from build123d import *

# Parameters (mm, degrees)
SKETCH1_W                    = 12
SKETCH1_H                    = 40
BOSS_EXTRUDE1_DEPTH          = 600
FILLET1_R                    = 12
SKETCH2_W                    = 1150
SKETCH2_H                    = 12
CUT_EXTRUDE1_DEPTH           = 2
FILLET2_R                    = 5
CUT_EXTRUDE2_REACH           = 14
SKETCH3_R                    = 4
F_4_0_4_DIAMETER_HOLE1_D     = 4
F_4_0_4_DIAMETER_HOLE1_DEPTH = 10
LPATTERN1_COUNT              = 4
LPATTERN1_PITCH              = 350
SKETCH6_W                    = 15
SKETCH6_H                    = 16
BOSS_EXTRUDE2_DEPTH          = 12
CUT_EXTRUDE6_REACH           = 17
SKETCH7_W                    = 2
SKETCH7_H                    = 12
FILLET3_R                    = 3


with BuildPart() as part:
    # Sketch1 → Boss-Extrude1 (new body, symmetric)
    with BuildSketch(Plane.XY):
        Rectangle(SKETCH1_W, SKETCH1_H)
    extrude(amount=BOSS_EXTRUDE1_DEPTH, both=True)

    # Fillet1
    fillet1_edges = [part.edges().sort_by_distance(p)[0] for p in [
        (0, -20, 600),
        (0, -20, -600),
        (0, 20, -600),
        (0, 20, 600),
    ]]
    fillet(fillet1_edges, radius=FILLET1_R)

    # Sketch2 → Cut-Extrude1 (cut)
    with BuildSketch(Plane(origin=(6, 0, 0), x_dir=(0, 0, -1), z_dir=(1, 0, 0))):
        with Locations((-25, 0)):
            Rectangle(SKETCH2_W, SKETCH2_H)
    extrude(amount=-CUT_EXTRUDE1_DEPTH, mode=Mode.SUBTRACT)

    # Fillet2
    fillet2_edges = [part.edges().sort_by_distance(p)[0] for p in [
        (5, 6, -550),
        (5, -6, -550),
    ]]
    fillet(fillet2_edges, radius=FILLET2_R)

    # Sketch3 → Cut-Extrude2 (cut, up to next)
    with BuildSketch(Plane(origin=(6, 0, 0), x_dir=(0, 0, -1), z_dir=(1, 0, 0)), mode=Mode.PRIVATE) as cut_extrude2_sk1:
        with Locations(Location((590, 0, 0), (0, 0, 90))):  # turned: the seam where the file's is
            Circle(SKETCH3_R)
    cut_extrude2_tool1 = extrude(cut_extrude2_sk1.sketch, amount=-CUT_EXTRUDE2_REACH, mode=Mode.PRIVATE) & part.part
    add(cut_extrude2_tool1.solids().sort_by_distance((6, 0, -590))[0], mode=Mode.SUBTRACT)

    # Ø4.0 (4) Diameter Hole1
    with Locations(Plane.ZY.offset(6)):
        with Locations((570, 0)):
            f_4_0_4_diameter_hole1 = Hole(F_4_0_4_DIAMETER_HOLE1_D / 2, depth=F_4_0_4_DIAMETER_HOLE1_DEPTH)

    # LPattern1: Ø4.0 (4) Diameter Hole1 ×4
    with Locations(*[(0, 0, -i * LPATTERN1_PITCH) for i in range(1, LPATTERN1_COUNT)]):
        add(f_4_0_4_diameter_hole1, mode=Mode.SUBTRACT)

    # Sketch6 → Boss-Extrude2 (add)
    with BuildSketch(Plane.ZY.offset(6)):
        with Locations((-607.5, 0)):
            Rectangle(SKETCH6_W, SKETCH6_H)
        with Locations((607.5, 0)):
            Rectangle(SKETCH6_W, SKETCH6_H)
    extrude(amount=-BOSS_EXTRUDE2_DEPTH)

    # Sketch7 → Cut-Extrude6 (cut, up to next)
    with BuildSketch(Plane(origin=(0, 0, 600), x_dir=(-1, 0, 0), z_dir=(0, 0, -1)), mode=Mode.PRIVATE) as cut_extrude6_sk1:
        with Locations((-5, 0)):
            Rectangle(SKETCH7_W, SKETCH7_H)
    cut_extrude6_tool1 = extrude(cut_extrude6_sk1.sketch, amount=-CUT_EXTRUDE6_REACH, mode=Mode.PRIVATE) & part.part
    add(cut_extrude6_tool1.solids().sort_by_distance((5, 0, 600))[0], mode=Mode.SUBTRACT)

    # Fillet3
    fillet3_edges = [part.edges().sort_by_distance(p)[0] for p in [
        (0, -8, 600),
        (0, 8, 600),
        (0, -8, -600),
        (0, 8, -600),
    ]]
    fillet(fillet3_edges, radius=FILLET3_R)


solid = part.part
CAD build for the part. Positions are in the model's coordinates, mm. Coordinates: 2 decimals unless noted, no trailing zeros. Order: outer loops, then holes, each group sorted by start corner. A loop starts at its lowest first (then second) coordinate and runs counter-clockwise, first axis right, second up. Notation, with made-up numbers: (-30.5, 29.25) -> (14.5, 29.25) arc R15 ccw to (14.5, 36.25) -> close; hole circle Ø4 at (-13.5, 49.5). An arc over 180 degrees is marked (long way). Answer in a Markdown table with one row per item.
1) Band-saw the part on B-B (z = -227.5). List the corners of the cut face in (x, y), and give its area (3 significant figures).
Check values:
| item | result |
|---|---|
| outline | (-6, -20) -> (6, -20) -> (6, -6) -> (4, -6) -> (4, 6) -> (6, 6) -> (6, 20) -> (-6, 20) -> close |
| area | 456 mm2 |
2) Drill centre lines: line 1 (Z direction, x = 3.25, y = 0.5); line 2 (Y direction, x = -0.5, z = 220); line 3 (X direction, y = 5.5, z = 72.5). Where is each one in solid material? Low to high.
Check values:
| item | result |
|---|---|
| line 1 | -615 to -593.97, -586.03 to -481.94, -478.06 to -131.94, -128.06 to 218.06, 221.94 to 568.06, 571.94 to 615 |
| line 2 | -20 to -2, 2 to 20 |
| line 3 | -6 to 4 |
3) Flat gauge pins, fed straight in: P1, Ø10, axis at y = 3.5, z = -384, coming from the +X side; P2, Ø3.5, axis at y = 0, z = -480, coming from the +X side; P3, Ø3, axis at x = -0.5, y = -13, coming from the -Z side; P4, Ø6, axis at x = 3, z = 607, coming from the +Y side. Where does each tip first touch, or does it go through?
Check values:
| item | result |
|---|---|
| P1 | x = 6 |
| P2 | through |
| P3 | z = -599.48 |
| P4 | y = 8 |
4) Band-saw the part on A-A (x = 1). List the corners of the cut face in (y, z), and give its area (3 significant figures).
Check values:
| item | result |
|---|---|
| outline | (-20, -588) arc R12 ccw to (-10.4, -599.76) arc R3 cw to (-8, -602.7) -> (-8, -615) -> (8, -615) -> (8, -602.7) arc R3 cw to (10.4, -599.76) arc R12 ccw to (20, -588) -> (20, 588) arc R12 ccw to (10.4, 599.76) arc R3 cw to (8, 602.7) -> (8, 615) -> (-8, 615) -> (-8, 602.7) arc R3 cw to (-10.4, 599.76) arc R12 ccw to (-20, 588) -> close; hole circle Ø8 at (0, -590); hole circle Ø4 at (0, -480); hole circle Ø4 at (0, -130); hole circle Ø4 at (0, 220); hole circle Ø4 at (0, 570) |
| area | 48,300 mm2 |
